Autodesk Inventor part; units mm, degrees
ref_plane "YZ Plane" through (0, 0, 0) normal (1, 0, 0) x (0, 1, 0)
ref_plane "XZ Plane" through (0, 0, 0) normal (0, 1, 0) x (-1, 0, 0)
ref_plane "XY Plane" through (0, 0, 0) normal (0, 0, 1) x (1, 0, 0)
sketch "Sketch1" plane through (0, 0, 0) normal (0, 1, 0) x (-1, 0, 0)
  line L0 (0, 0) -> (-60, 0)
  line L1 (-60, 0) -> (-60, -60)
  line L2 (-60, -60) -> (0, -60)
  line L3 (0, -60) -> (0, 0)
  dimension "d0" = 60
  dimension "d1" = 60
extrude "Extrusion1" add sketch "Sketch1" along normal blind 3
sketch "Sketch2" plane through (0, 0, 0) normal (0, 0, 1) x (1, 0, 0)
  line L0 (60, 0) -> (0, 0)
  line L1 (0, 0) -> (60, 0)
  line L2 (60, 0) -> (60, 60)
  line L3 (60, 60) -> (0, 60)
  line L4 (0, 60) -> (0, 0)
  line L5 (0, 0) -> (60, 0)
  line L6 (0, 0) -> (60, 0)
  line L7 (60, 0) -> (60, 3)
  line L8 (0, 3) -> (60, 3)
  line L9 (0, 0) -> (0, 3)
  dimension "d4" = 60
  dimension "d5" = 60
extrude "Extrusion2" add sketch "Sketch2" against normal blind 3 contours L8 L4 L3 L2
properties part number "T4788-SWERVE-004-BRACKET"
For this review, take the finished solid that the model builds, in its own axes (mm). A direction names the side the tool comes from. Give positions to 0.01 mm unless a question says otherwise; leave off trailing zeros. Order: outer loops, then holes, each group sorted by start corner. A loop starts at its lowest first (then second) coordinate and runs counter-clockwise, first axis right, second up. Notation, with made-up numbers: M 79.5,-28.75 L 89.5,-28.75 A20 cw 89.5,-15.75 Z; hole C -18,76.25 d11. An arc over 180 degrees is marked long. Answer in a Markdown table with one row per item. Add a question column.
(1) For pin 1 (3 mm diameter, centred on x = 24.5, y = 23.5, fed in from +Z); pin 2 (3 mm diameter, centred on x = 49, y = 43, fed in from -Z), all flat-tipped, find the tip position at first contact; note any pin that passes through.
(2) For faces 1 (the face through (30, 60, -1)), 2 (the face through (30, 32, -3)), list the 3-axis set-ups (+Z, -Z, +X, -X, +Y, -Y) from which the entire face can be reached by the end or side of a thin tool; tool diameter is ignored.
(3) Consider section B-B on y = 28. State the section outline as (x, z) points.
(4) Consider section A-A on x = 6.5. State the section outline as (y, z) points.
(5) Consider section C-C on z = -36.5. State the section outline as (x, y) points.
(6) Wall thickness on probe 1 along Y at (x, z) = (20.5, -47); probe 2 along Z at (x, y) = (6, 19.5): over which ranges is each line inside the solid? List them lowest first. Write a range as [from, to].
Evaluation:
| question | item | result |
|---|---|---|
| 1 | pin 1 | stops at z = 0 |
| 1 | pin 2 | stops at z = -3 |
| 2 | face 1 | +Z, -Z, +X, -X, +Y |
| 2 | face 2 | -Z, +X, -X, +Y |
| 3 | outline | M 0,-3 L 60,-3 L 60,0 L 0,0 Z |
| 4 | outline | M 0,-60 L 3,-60 L 3,-3 L 60,-3 L 60,0 L 0,0 Z |
| 5 | outline | M 0,0 L 60,0 L 60,3 L 0,3 Z |
| 6 | probe 1 | y = [0, 3] |
| 6 | probe 2 | z = [-3, 0] |
